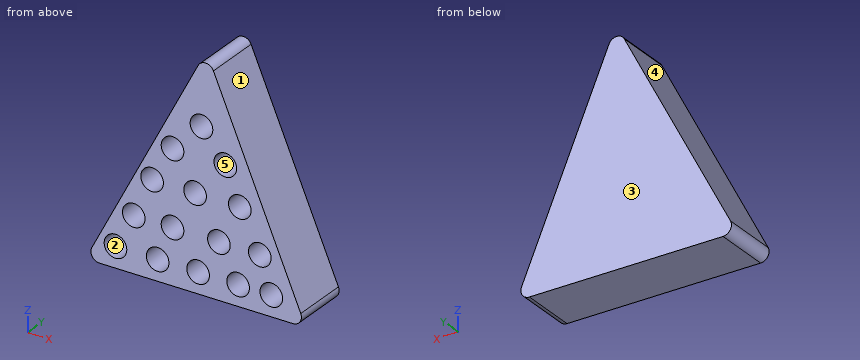
from build123d import *

# Parameters (mm, degrees)
F1_DEPTH = 25.4
F2_R     = 5.08
F3_DEPTH = 22.86


with BuildPart() as f1:
    # F0 (on Front) → F1 (new body)
    with BuildSketch(Plane.XZ):
        with BuildLine():
            ThreePointArc((3.163813, 68.164682), (-0.191852, 70.466917), (-3.712345, 68.425619))
            Line((-3.712345, 68.425619), (-51.374926, -22.691637))
            ThreePointArc((-51.374926, -22.691637), (-51.258083, -26.430894), (-47.998911, -28.267599))
            Line((-47.998911, -28.267599), (38.843141, -28.267599))
            ThreePointArc((38.843141, -28.267599), (42.025141, -26.553065), (42.343284, -22.952574))
            Line((42.343284, -22.952574), (3.163813, 68.164682))
        make_face()
    extrude(amount=F1_DEPTH)

    # F2 (on face) → F3 (cut)
    with BuildSketch(Plane.XZ.offset(25.4)):
        with Locations((-24.346719, 14.035167)):
            Circle(F2_R)
        with Locations((-15.180895, 29.884405)):
            Circle(F2_R)
        with Locations((-2.195979, 43.060273)):
            Circle(F2_R)
        with Locations((-3.712345, -18.999988)):
            Circle(F2_R)
        with Locations((14.226123, -18.999988)):
            Circle(F2_R)
        with Locations((29.120583, -18.999988)):
            Circle(F2_R)
        with Locations((-21.864308, -18.999988)):
            Circle(F2_R)
        with Locations((-40.768821, -18.999988)):
            Circle(F2_R)
        with Locations((-32.557767, -3.532661)):
            Circle(F2_R)
        with Locations((-15.180895, -3.532661)):
            Circle(F2_R)
        with Locations((5.633163, -3.532661)):
            Circle(F2_R)
        with Locations((23.964809, -3.532661)):
            Circle(F2_R)
        with Locations((14.989941, 14.035167)):
            Circle(F2_R)
        with Locations((-5.060299, 14.035167)):
            Circle(F2_R)
        with Locations((8.497481, 29.884405)):
            Circle(F2_R)
    extrude(amount=-F3_DEPTH, mode=Mode.SUBTRACT)


solid = f1.part
The listing builds one solid part. Answer for the finished solid, in the listing's coordinates (mm). Face numbers are marked on the shaded views. A direction names the side the tool comes from. Give positions to 0.01 mm unless a question says otherwise; leave off trailing zeros. Order: outer loops, then holes, each group sorted by start corner. A loop starts at its lowest first (then second) coordinate and runs counter-clockwise, first axis right, second up. Notation, with made-up numbers: (-10, 85.25) -> (16, 85.25) arc R35 cw to (16, 120.25) -> close; hole circle Ø2 at (50.5, 80.25). An arc over 180 degrees is marked (long way). Put each result on its own line as item: value.
Item 1: A cutting plane is placed at A-A on y = -15. Count the separate pieces of the cut face and the enclosed holes in it, plus the area to 3 significant figures.
Established:
separate pieces: 1
enclosed holes: 15
area: 3,890 mm^2
Item 2: For the marked faces 1 and 2, determine the directions among +Z, -Z, +X, -X, +Y, -Y from which every point of the face is accessible in a straight line to the end or side of a thin tool.
Established:
face 1: +Z, +X, +Y, -Y
face 2: -Y
Item 3: A cutting plane is placed at C-C on x = 31. Give the vertices of the cut face in (y, z).
Established:
outline: (-25.4, -28.27) -> (0, -28.27) -> (0, 3.43) -> (-25.4, 3.43) -> (-25.4, -14.28) -> (-2.54, -14.28) -> (-2.54, -23.72) -> (-25.4, -23.72) -> close
Item 4: Given P1, Ø1.5, axis at y = -17.5, z = 22.5, coming from the +X side; P2, Ø3, axis at y = -16, z = -6, coming from the +X side; P3, Ø1.5, axis at y = -14.5, z = 26, coming from the -X side, each flat-ended and moving along its own axis, determine where each tip first touches the part or whether it passes through.
Established:
P1: stops at x = 23.12
P2: stops at x = 35.7
P3: stops at x = -26.3
Item 5: Straight lines are drawn through the part: line 1 (Z direction, x = -25, y = -6.5); line 2 (X direction, y = -11.5, z = 27.5); line 3 (Z direction, x = -6, y = -18.75). For each, find the intervals that lie inside material, in ascending order.
Established:
line 1: z = -28.27 to -23, -15 to 9, 19.07 to 27.73
line 2: x = -25.12 to -19.67, -10.7 to 4.01, 12.98 to 20.65
line 3: z = -28.27 to -23.54, -14.46 to 9.04, 19.03 to 39.69, 46.43 to 64.05
Item 6: A cutting plane is placed at D-D on z = -16.5. Give the vertices of the cut face in (x, y).
Established:
outline: (-48.14, -25.4) -> (-45.19, -25.4) -> (-45.19, -2.54) -> (-36.35, -2.54) -> (-36.35, -25.4) -> (-26.29, -25.4) -> (-26.29, -2.54) -> (-17.44, -2.54) -> (-17.44, -25.4) -> (-8.13, -25.4) -> (-8.13, -2.54) -> (0.71, -2.54) -> (0.71, -25.4) -> (9.8, -25.4) -> (9.8, -2.54) -> (18.65, -2.54) -> (18.65, -25.4) -> (24.7, -25.4) -> (24.7, -2.54) -> (33.54, -2.54) -> (33.54, -25.4) -> (39.57, -25.4) -> (39.57, 0) -> (-48.14, 0) -> close
Item 7: A cutting plane is placed at B-B on z = 11. Give the vertices of the cut face in (x, y).
Established:
outline: (-33.75, -25.4) -> (-28.42, -25.4) -> (-28.42, -2.54) -> (-20.27, -2.54) -> (-20.27, -25.4) -> (-9.13, -25.4) -> (-9.13, -2.54) -> (-0.99, -2.54) -> (-0.99, -25.4) -> (10.92, -25.4) -> (10.92, -2.54) -> (19.06, -2.54) -> (19.06, -25.4) -> (27.74, -25.4) -> (27.74, 0) -> (-33.75, 0) -> close
Item 8: For a pull along Z with two mould halves and no side action, classify the marked faces 3, 4 and 5 as released by +Z, released by -Z, zero draft, split by the parting line, or undercut.
Established:
face 3: zero draft
face 4: released by +Z
face 5: undercut
